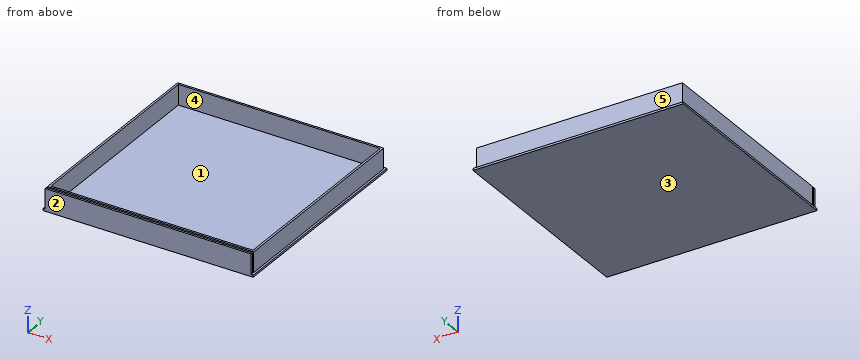
Autodesk Fusion 360 part; units mm, degrees
sketch "Szkic5" plane through (0, 0, 0) normal (0, 0, 1) x (1, 0, 0)
  line L0 (-100, 100) -> (100, 100)
  line L1 (100, 100) -> (100, -100)
  line L2 (100, -100) -> (-100, -100)
  line L3 (-100, -100) -> (-100, 100)
  line L4 (-102, 102) -> (102, 102)
  line L5 (102, 102) -> (102, -102)
  line L6 (102, -102) -> (-102, -102)
  line L7 (-102, -102) -> (-102, 102)
  line L8 (-104, 104) -> (104, 104)
  line L9 (104, 104) -> (104, -104)
  line L10 (104, -104) -> (-104, -104)
  line L11 (-104, -104) -> (-104, 104)
  line L12 (-106, 106) -> (106, 106)
  line L13 (106, 106) -> (106, -106)
  line L14 (106, -106) -> (-106, -106)
  line L15 (-106, -106) -> (-106, 106)
  line L16 (-104, -104) -> (-104, -106)
  line L17 (104, -104) -> (104, -106)
  line L18 (102, -102) -> (102, -104)
  line L19 (-102, -102) -> (-102, -104)
  line L20 (-102, -104) -> (-102, -106)
  line L21 (104, -104) -> (104, -106)
  line L22 (102, -104) -> (102, -106)
  dimension "d31" = 2
  dimension "d32" = 2
  dimension "d33" = 2
  dimension "d34" = 2
  dimension "d35" = 2
  dimension "d36" = 2
  dimension "d37" = 2
  dimension "d38" = 2
  dimension "d39" = 2
  dimension "d40" = 2
  dimension "d41" = 2
  dimension "d42" = 2
extrude "Wyciągnięcie proste15" add sketch "Szkic5" against normal blind 2 contours L0 L1 L2 L3 | L4 L5 L7 L8 L9 L10 L11 L18 L19 | L4 L5 L6 L7 | L6 L10 L18 L19 | L10 L14 L16 L20 | L10 L14 L20 L22 | L10 L14 L17 L21 L22 | L8 L9 L11 L12 L13 L14 L15 L16 L17 L21
extrude "Wyciągnięcie proste16" add sketch "Szkic5" along normal blind 15 contours L4 L5 L6 L7
extrude "Wyciągnięcie proste17" add sketch "Szkic5" along normal blind 15 contours L10 L14 L16 L20 | L10 L14 L20 L22 | L10 L14 L17 L21 L22
extrude "Wyciągnięcie proste18" cut sketch "Szkic5" against normal blind 2 contours L8 L9 L11 L12 L13 L14 L15 L16 L17 L21
extrude "Extrude19" cut sketch "Szkic5" along normal blind 15 contours L10 L14 L16 L20 | L10 L14 L17 L21 L22
extrude "Extrude20" add 2 faces at (-33.3333, -101.3333, 15) (-34, -105.3333, 15) along direction (0, 0, 1) blind 5
Can you work these out from the model? Positions are in its coordinate system, mm. Face numbers are marked on the shaded views. A direction names the side the tool comes from. Give positions to 0.01 mm unless a question says otherwise; leave off trailing zeros. Write each loop counter-clockwise with the first axis right and the second up, starting at its lowest first coordinate (ties: lowest second). Pieces come first, ordered by that corner, then holes. Notation, with made-up numbers: (61, -3) -> (102, -3) arc R19 cw to (102, 27) -> close; hole circle Ø10 at (43.25, 36.25). An arc over 180 degrees is marked (long way). Answer as a JSON object with one key per item and string values. Group by question number.
Item 1: Suppose I cut it at C-C (x = 63). Please give me the cut outline in (y, z).
Item 2: I'm going to push flat-ended pins straight in: P1, Ø1, axis at x = -63, z = 11, coming from the +Y side; P2, Ø0.6, axis at y = -105, z = 13.5, coming from the -X side; P3, Ø6, axis at x = -61.5, y = 48, coming from the +Z side. Where does each tip first touch, or does it pass through?
Item 3: Suppose I cut it at A-A (z = 16.25). Please give me the cut outline in (x, y), plus the area to 3 significant figures.
Item 4: Please list where these lines run through material, in increasing order: line 1 (Y direction, x = 25.5, z = 7.5); line 2 (X direction, y = -68, z = 7.5); line 3 (Z direction, x = 32, y = 33). Write a range as [from, to].
Item 5: Suppose I cut it at B-B (y = -51.5). Please give me the cut outline in (x, z).
Item 6: We'd pull the mould along Y, two halves only. Please class the marked faces 3, 4 and 5: +Y half, -Y half, draft (parallel to the pull), parting line (faces both ways), or undercut.
Item 7: For the marked faces 1 and 2, which set-ups out of +Z, -Z, +X, -X, +Y, -Y let a thin tool reach every point of the face, with its end or its side?
Findings:
{
 "1": {"outline": "(-106, -2) -> (104, -2) -> (104, 0) -> (102, 0) -> (102, 20) -> (100, 20) -> (100, 0) -> (-100, 0) -> (-100, 20) -> (-102, 20) -> (-102, 0) -> (-104, 0) -> (-104, 20) -> (-106, 20) -> close"},
 "2": {"P1": "stops at y = 102", "P2": "stops at x = -102", "P3": "stops at z = 0"},
 "3": {"outline": "(-102, -106) -> (102, -106) -> (102, -104) -> (-102, -104) -> close; (-102, -102) -> (102, -102) -> (102, 102) -> (-102, 102) -> close; hole (-100, -100) -> (100, -100) -> (100, 100) -> (-100, 100) -> close", "area": "2,020 mm²"},
 "4": {"line 1": "y = [-106, -104], [-102, -100], [100, 102]", "line 2": "x = [-102, -100], [100, 102]", "line 3": "z = [-2, 0]"},
 "5": {"outline": "(-104, -2) -> (104, -2) -> (104, 0) -> (102, 0) -> (102, 20) -> (100, 20) -> (100, 0) -> (-100, 0) -> (-100, 20) -> (-102, 20) -> (-102, 0) -> (-104, 0) -> close"},
 "6": {"face 3": "draft", "face 4": "undercut", "face 5": "+Y half"},
 "7": {"face 1": "+Z", "face 2": "+Z, -Z, +X, -X, -Y"}
}
